Design review of the part shown in the three views and the two pictorial views. Dimensions are in mm from the part's minimum x, y and z. Give positions to 0.01 mm unless a question says otherwise; leave off trailing zeros. Loops run counter-clockwise (first coordinate to the right, second up) from the corner with the lowest first, then second, coordinate; pieces in that order, holes last. Notation, with made-up numbers: (83, 60.25) -> (121, 60.25) arc R17 ccw to (121, 79.25) -> close; hole circle Ø11 at (23.25, -8). An arc over 180 degrees is marked (long way). Use CSV: the item, a comma, the result in double quotes. Start each with the question number.
Item 1: We need section B-B (x = 14). State the section outline as (y, z) points.
Item 2: Clearance check with flat-ended pins moving along their axes: pin 1 (10 mm diameter, centred on y = 187.5, z = 3.5, fed in from +X); pin 2 (2 mm diameter, centred on x = 75, z = 4.5, fed in from +Y); pin 3 (2 mm diameter, centred on x = 111, z = 6.5, fed in from +Y). State where each tip first meets the part, or that it passes through.
Item 3: We need section A-A (z = 14.25). State the section outline as (x, y) points, plus the area to 3 significant figures.
Item 4: We need section C-C (y = 175). State the section outline as (x, z) points, plus the area to 3 significant figures.
Item 5: Wall thickness on line 1 along Y through (x, z) = (127.5, 16.75); line 2 along Y through (x, z) = (59, 13); line 3 along X through (y, z) = (136, 10): over which ranges is each line inside the solid? List them lowest first. Write a range as from..to.
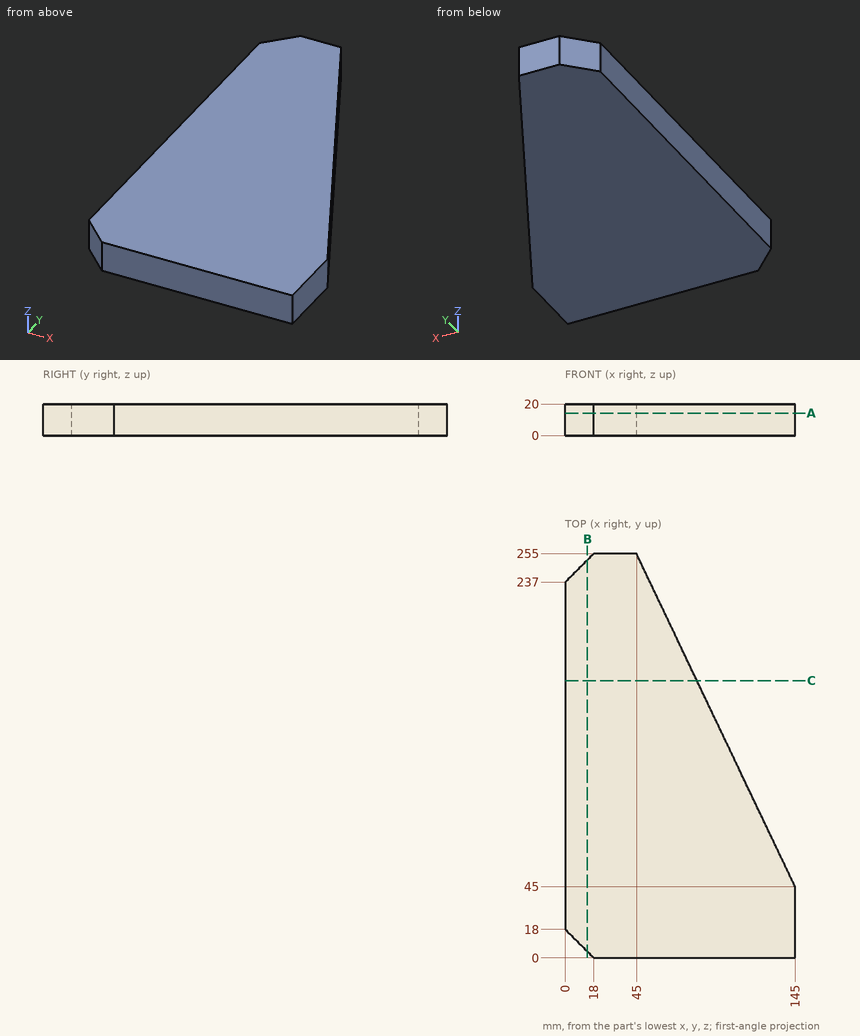
Results found:
1,outline,"(4, 0) -> (251, 0) -> (251, 20) -> (4, 20) -> close"
2,pin 1,"x = 79.52"
2,pin 2,"y = 194.1"
2,pin 3,"y = 118.5"
3,outline,"(0, 18) -> (18, 0) -> (145, 0) -> (145, 45) -> (45, 255) -> (18, 255) -> (0, 237) -> close"
3,area,"26,200 mm²"
4,outline,"(0, 0) -> (83.1, 0) -> (83.1, 20) -> (0, 20) -> close"
4,area,"1,660 mm²"
5,line 1,"0..81.75"
5,line 2,"0..225.6"
5,line 3,"0..101.67"
